from build123d import *

# Parameters (mm, degrees)
SKETCH008_W     = 44.58321
SKETCH008_H     = 44.7
PAD006_DEPTH    = 126.628014
THICKNESS_T     = 1.5
SKETCH009_W     = 12
SKETCH009_H     = 8.605206
SKETCH009_H_2   = 8.931469
PAD007_DEPTH    = 8
SKETCH010_W     = 12.1
SKETCH010_H     = 8.476139
SKETCH010_W_2   = 12
SKETCH010_H_2   = 8.882789
PAD008_DEPTH    = 5
SKETCH014_W     = 11.6
SKETCH014_H     = 20.6
POCKET003_DEPTH = 5
FILLET_R        = 4.8


with BuildPart() as part:
    # Sketch008 (on Face1 of ShapeBinder002) → Pad006 (new body)
    with BuildSketch(Plane(origin=(0, -63.568756, 0), x_dir=(0, 0, -1), z_dir=(0, -1, 0))):
        with Locations((-79.071486, 9.742272)):
            Rectangle(SKETCH008_W, SKETCH008_H)
    extrude(amount=-PAD006_DEPTH)

    # Thickness
    thickness_openings = [part.faces().sort_by_distance(p)[0] for p in [
        (9.742272, -0.254749, 56.779881),
    ]]
    offset(amount=THICKNESS_T, openings=thickness_openings)

    # Sketch009 (on Face5 of Thickness) → Pad007 (join)
    with BuildSketch(Plane.YZ.offset(-12.607728)):
        with Locations((-37.374453, 61.145227)):
            Rectangle(SKETCH009_W, SKETCH009_H)
        with Locations((33.398816, 61.123247)):
            Rectangle(SKETCH009_W, SKETCH009_H_2)
    extrude(amount=PAD007_DEPTH)

    # Sketch010 (on Face1 of Pad007) → Pad008 (join)
    with BuildSketch(Plane(origin=(32.092272, 0, 0), x_dir=(0, -1, 0), z_dir=(-1, 0, 0))):
        with Locations((-33.333797, 61.228186)):
            Rectangle(SKETCH010_W, SKETCH010_H)
        with Locations((37.319737, 61.147633)):
            Rectangle(SKETCH010_W_2, SKETCH010_H_2)
    extrude(amount=PAD008_DEPTH)

    # Sketch014 (on Face45 of Pad008) → Pocket003 (cut)
    with BuildSketch(Plane.XY.offset(102.863091)):
        with Locations((-5.087287, -4.135811)):
            Rectangle(SKETCH014_W, SKETCH014_H)
    extrude(amount=-POCKET003_DEPTH, mode=Mode.SUBTRACT)

    # Fillet
    fillet_edges = [part.edges().sort_by_distance(p)[0] for p in [
        (32.092272, -37.319737, 65.589027),
        (32.092272, 33.333797, 65.466255),
        (-12.607728, -37.374453, 65.44783),
        (-12.607728, 33.398816, 65.588982),
    ]]
    fillet(fillet_edges, radius=FILLET_R)


solid = part.part
The model under review builds one solid part; all positions refer to its coordinate system, in mm. A direction names the side the tool comes from. Round coordinates to 2 decimals unless told otherwise and drop trailing zeros. Loops run counter-clockwise (first coordinate to the right, second up) from the corner with the lowest first, then second, coordinate; pieces in that order, holes last. Notation, with made-up numbers: M 43,49 L 60,49 A8 cw 60,61 Z; hole C -2.75,33.5 d6. An arc over 180 degrees is marked long. Answer as CSV lines item,"result".
1. Draft analysis for pull direction Z (two halves, no side actions). For faces 3 (the face through (-9, 33, 56.658)), 4 (the face through (30.65, -37.4, 66.96)), 5 (the face through (30, -31.32, 62)), state which applies: pulls with the +Z half, pulls with the -Z half, needs draft (parallel to the pull), parting line crosses it, or undercut.
Outcome:
face 3,"pulls with the -Z half"
face 4,"undercut"
face 5,"needs draft"
2. We need section D-D (z = 93.5). Give the boundary of the cut face in (x, y), plus the area to 3 significant figures.
Outcome:
outline,"M -14.11,-63.57 A1.5 ccw -12.61,-65.07 L 32.09,-65.07 A1.5 ccw 33.59,-63.57 L 33.59,63.06 A1.5 ccw 32.09,64.56 L -12.61,64.56 A1.5 ccw -14.11,63.06 Z; hole M -12.61,-63.57 L 32.09,-63.57 L 32.09,63.06 L -12.61,63.06 Z"
area,"521 mm2"
3. We need section A-A (z = 60.5). Give the boundary of the cut face in (x, y).
Outcome:
outline,"M -14.11,-63.57 A1.5 ccw -12.61,-65.07 L 32.09,-65.07 A1.5 ccw 33.59,-63.57 L 33.59,63.06 A1.5 ccw 32.09,64.56 L -12.61,64.56 A1.5 ccw -14.11,63.06 Z; hole M -12.61,-63.57 L 32.09,-63.57 L 32.09,-43.32 L 27.09,-43.32 L 27.09,-31.32 L 32.09,-31.32 L 32.09,27.28 L 27.09,27.28 L 27.09,39.38 L 32.09,39.38 L 32.09,63.06 L -12.61,63.06 L -12.61,39.4 L -4.61,39.4 L -4.61,27.4 L -12.61,27.4 L -12.61,-31.37 L -4.61,-31.37 L -4.61,-43.37 L -12.61,-43.37 Z"
4. For faces 1 (the face through (-4.608, -37, 61)), 2 (the face through (10, -65.069, 79)), list the 3-axis set-ups (+Z, -Z, +X, -X, +Y, -Y) from which the entire face can be reached by the end or side of a thin tool; tool diameter is ignored.
Outcome:
face 1,"-Z"
face 2,"+Z, -Z, +X, -X, -Y"
5. We need section C-C (x = 23). Give the boundary of the cut face in (y, z).
Outcome:
outline,"M -65.07,56.78 L -63.57,56.78 L -63.57,101.36 L 63.06,101.36 L 63.06,56.78 L 64.56,56.78 L 64.56,101.36 A1.5 ccw 63.06,102.86 L -63.57,102.86 A1.5 ccw -65.07,101.36 Z"
6. We need section B-B (y = -25). Give the boundary of the cut face in (x, z), plus the area to 3 significant figures.
Outcome:
outline,"M -14.11,56.78 L -12.61,56.78 L -12.61,101.36 L 32.09,101.36 L 32.09,56.78 L 33.59,56.78 L 33.59,101.36 A1.5 ccw 32.09,102.86 L -12.61,102.86 A1.5 ccw -14.11,101.36 Z"
area,"204 mm2"
7. Insertion check: pin 1 Ø1.5 at (x, y) = (29, 34) entering from -Z; pin 2 Ø0.8 at (y, z) = (-5, 102) entering from +X; pin 3 Ø13.5 at (x, y) = (20, 10.5) entering from -Z; pin 4 Ø1.6 at (x, z) = (-8, 102) entering from +Y. Each pin has a flat end and moves straight along its axis. Give the tip position at first contact, or say it passes through.
Outcome:
pin 1,"stops at z = 56.99"
pin 2,"stops at x = 33.57"
pin 3,"stops at z = 101.36"
pin 4,"stops at y = 64.56"
8. To check wall thickness, follow L1, parallel to Y at x = -9, z = 96.5; L2, parallel to X at y = 38, z = 60; L3, parallel to X at y = -25, z = 74. State the ranges of each line that lie inside material, in increasing order. Write a range as [from, to].
Outcome:
L1,"y = [-65.07, -63.57], [63.06, 64.56]"
L2,"x = [-14.11, -4.61], [27.09, 33.59]"
L3,"x = [-14.11, -12.61], [32.09, 33.59]"
